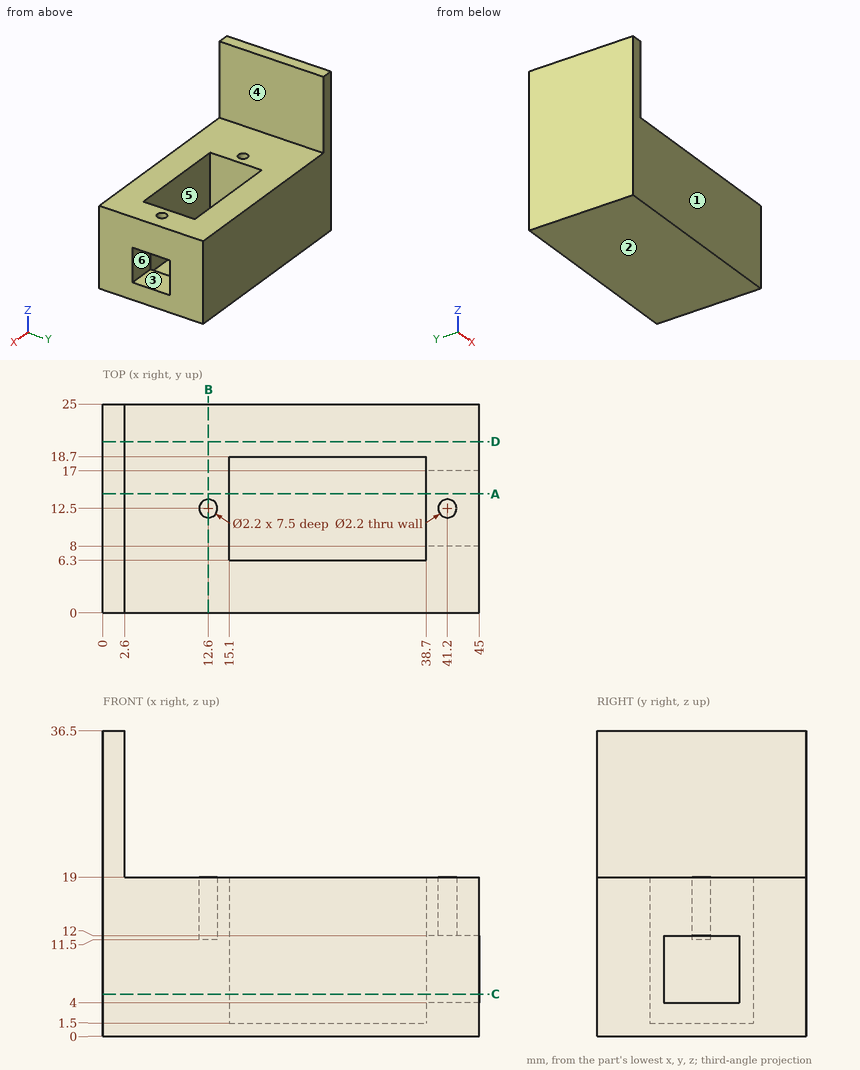
Could you check a few things on this drawing? It's one solid part, dimensions in mm from its lowest x, y, z. A direction names the side the tool comes from. Coordinates: 2 decimals unless noted, no trailing zeros. Loops run counter-clockwise (first coordinate to the right, second up) from the corner with the lowest first, then second, coordinate; pieces in that order, holes last. Notation, with made-up numbers: (67.25, -23) - (114.25, -23) arc R23 cw to (114.25, 3) - close; hole circle Ø10 at (21.25, -4). An arc over 180 degrees is marked (long way). Return JSON: item names as keys, results as strings. Group by question number.
Item 1: I need wall thicknesses on line 1 (Y direction, x = 12.6, z = 16.75); line 2 (Y direction, x = 17, z = 14.5); line 3 (X direction, y = 17.25, z = 10.5). Which ranges of each line are inside material? Lowest first, please. Write a range as from..to.
Item 2: Will these pins go through, and if not, where does the flat tip stop? P1, Ø3, axis at x = 40.5, y = 12.5, coming from the +Z side; P2, Ø14, axis at y = 13, z = 27, coming from the +X side.
Item 3: If we section it at B-B on x = 12.6: Write out the boundary of the cut face in (y, z).
Item 4: If we section it at A-A on y = 14.25: Write out the boundary of the cut face in (x, z), and give its area (3 significant figures).
Item 5: On a 3-axis mill with a long thin cutter (end or side, diameter ignored), from which of +Z, -Z, +X, -X, +Y, -Y can I reach the whole of each face in a straight line? I mean the marked faces 4, 5 and 6. Say none if no direction works.
Item 6: If we section it at D-D on y = 20.5: Write out the boundary of the cut face in (x, z).
Item 7: If we section it at C-C on z = 5: Write out the boundary of the cut face in (x, y), and give its area (3 significant figures).
Item 8: We'd pull the mould along Y, two halves only. Please class the marked faces 1, 2 and 3: +Y half, -Y half, draft (parallel to the pull), parting line (faces both ways), or undercut.
Calculated:
{
 "1": {"line 1": "y = 0..11.4, 13.6..25", "line 2": "y = 0..6.3, 18.7..25", "line 3": "x = 0..15.1, 38.7..45"},
 "2": {"P1": "stops at z = 19", "P2": "stops at x = 2.6"},
 "3": {"outline": "(0, 0) - (25, 0) - (25, 19) - (13.6, 19) - (13.6, 11.5) - (11.4, 11.5) - (11.4, 19) - (0, 19) - close"},
 "4": {"outline": "(0, 0) - (45, 0) - (45, 4) - (38.7, 4) - (38.7, 1.5) - (15.1, 1.5) - (15.1, 19) - (2.6, 19) - (2.6, 36.5) - (0, 36.5) - close; (38.7, 12) - (45, 12) - (45, 19) - (38.7, 19) - close", "area": "437 mm^2"},
 "5": {"face 4": "+Z, +X, +Y, -Y", "face 5": "+Z", "face 6": "+X"},
 "6": {"outline": "(0, 0) - (45, 0) - (45, 19) - (2.6, 19) - (2.6, 36.5) - (0, 36.5) - close"},
 "7": {"outline": "(0, 0) - (45, 0) - (45, 8) - (38.7, 8) - (38.7, 6.3) - (15.1, 6.3) - (15.1, 18.7) - (38.7, 18.7) - (38.7, 17) - (45, 17) - (45, 25) - (0, 25) - close", "area": "776 mm^2"},
 "8": {"face 1": "-Y half", "face 2": "draft", "face 3": "undercut"}
}
